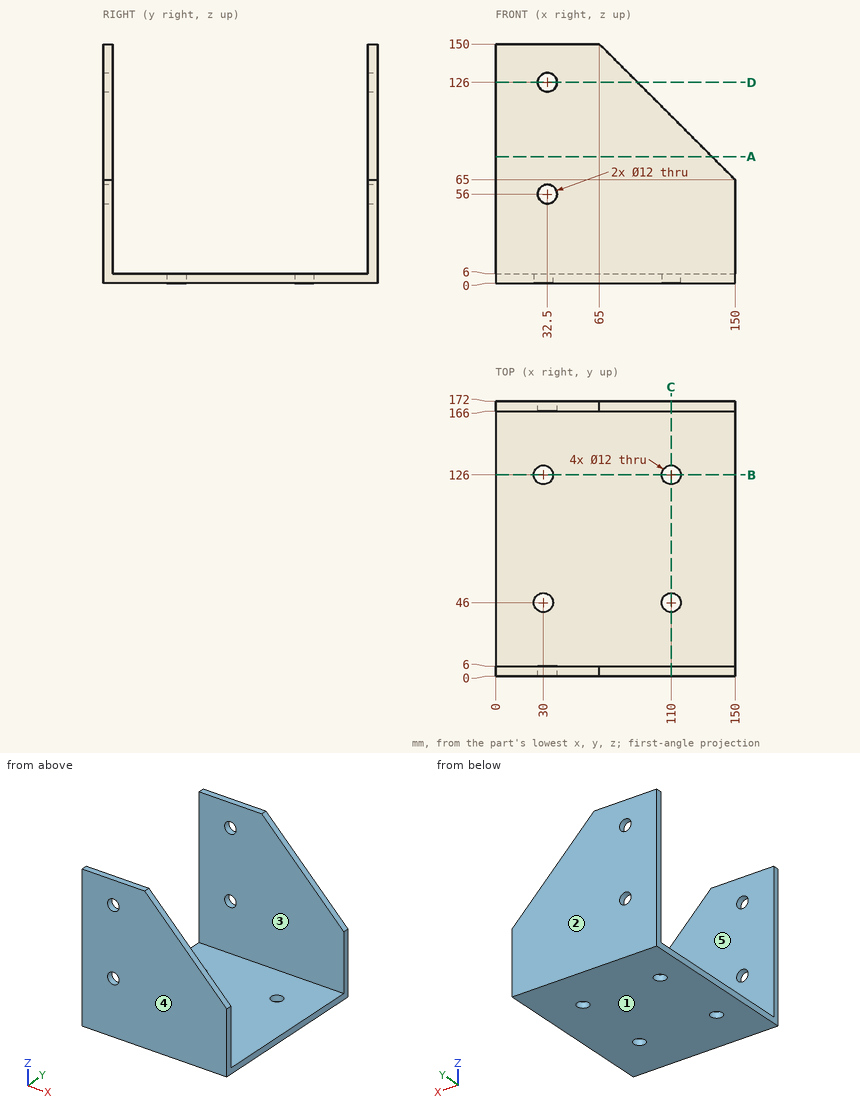
Verification items for this drawing (mm, ordinates from the low corner). A direction names the side the tool comes from. Give positions to 0.01 mm unless a question says otherwise; leave off trailing zeros. Write each loop counter-clockwise with the first axis right and the second up, starting at its lowest first coordinate (ties: lowest second). Pieces come first, ordered by that corner, then holes. Notation, with made-up numbers: (13.25, 24.25) - (39.25, 24.25) arc R26 ccw to (39.25, 43.25) - close; hole circle Ø8 at (-31.75, 54). An arc over 180 degrees is marked (long way). Answer as a JSON object with one key per item and string values. Group by question number.
1) Access from +Z, -Z, +X, -X, +Y, -Y to the whole of each face (thin tool, end or side, straight path). Record for the marked faces 4 and 5.
2) Thickness scan on probe 1 along Y at (x, z) = (30, 3); probe 2 along X at (y, z) = (126, 2.7); probe 3 along Z at (x, y) = (32.5, 4.1). Record the ranges inside material, lowest first. Write a range as from..to.
3) Sectioned sample at B-B (y = 126). Record the cut outline in (x, z), then the cut area to 3 significant figures.
4) Depth check by flat-ended pin: P1, Ø9.5, axis at x = 30, y = 126, coming from the -Z side; P2, Ø14, axis at x = 110, y = 46, coming from the +Z side. Enter the tip coordinate at first touch or a pass-through.
5) Sectioned sample at D-D (z = 126). Record the cut outline in (x, y), then the cut area to 3 significant figures.
6) Sectioned sample at C-C (x = 110). Record the cut outline in (y, z), then the cut area to 3 significant figures.
7) Release check for a two-part mould opening along Y. For the marked faces 1, 2 and 3 record: pulls with the +Y half, pulls with the -Y half, needs draft (parallel to the pull), parting line crosses it, or undercut.
8) Sectioned sample at A-A (z = 79.5). Record the cut outline in (x, y), then the cut area to 3 significant figures.
Geometry results:
{
 "1": {"face 4": "+Z, -Z, +X, -X, -Y", "face 5": "+Z, +X, -X"},
 "2": {"probe 1": "y = 0..40, 52..120, 132..172", "probe 2": "x = 0..24, 36..104, 116..150", "probe 3": "z = 0..50, 62..120, 132..150"},
 "3": {"outline": "(0, 0) - (24, 0) - (24, 6) - (0, 6) - close; (36, 0) - (104, 0) - (104, 6) - (36, 6) - close; (116, 0) - (150, 0) - (150, 6) - (116, 6) - close", "area": "756 mm^2"},
 "4": {"P1": "passes through", "P2": "stops at z = 6"},
 "5": {"outline": "(0, 0) - (26.5, 0) - (26.5, 6) - (0, 6) - close; (0, 166) - (26.5, 166) - (26.5, 172) - (0, 172) - close; (38.5, 0) - (89, 0) - (89, 6) - (38.5, 6) - close; (38.5, 166) - (89, 166) - (89, 172) - (38.5, 172) - close", "area": "924 mm^2"},
 "6": {"outline": "(0, 0) - (40, 0) - (40, 6) - (6, 6) - (6, 105) - (0, 105) - close; (52, 0) - (120, 0) - (120, 6) - (52, 6) - close; (132, 0) - (172, 0) - (172, 105) - (166, 105) - (166, 6) - (132, 6) - close", "area": "2,080 mm^2"},
 "7": {"face 1": "needs draft", "face 2": "pulls with the +Y half", "face 3": "undercut"},
 "8": {"outline": "(0, 0) - (135.5, 0) - (135.5, 6) - (0, 6) - close; (0, 166) - (135.5, 166) - (135.5, 172) - (0, 172) - close", "area": "1,630 mm^2"}
}
